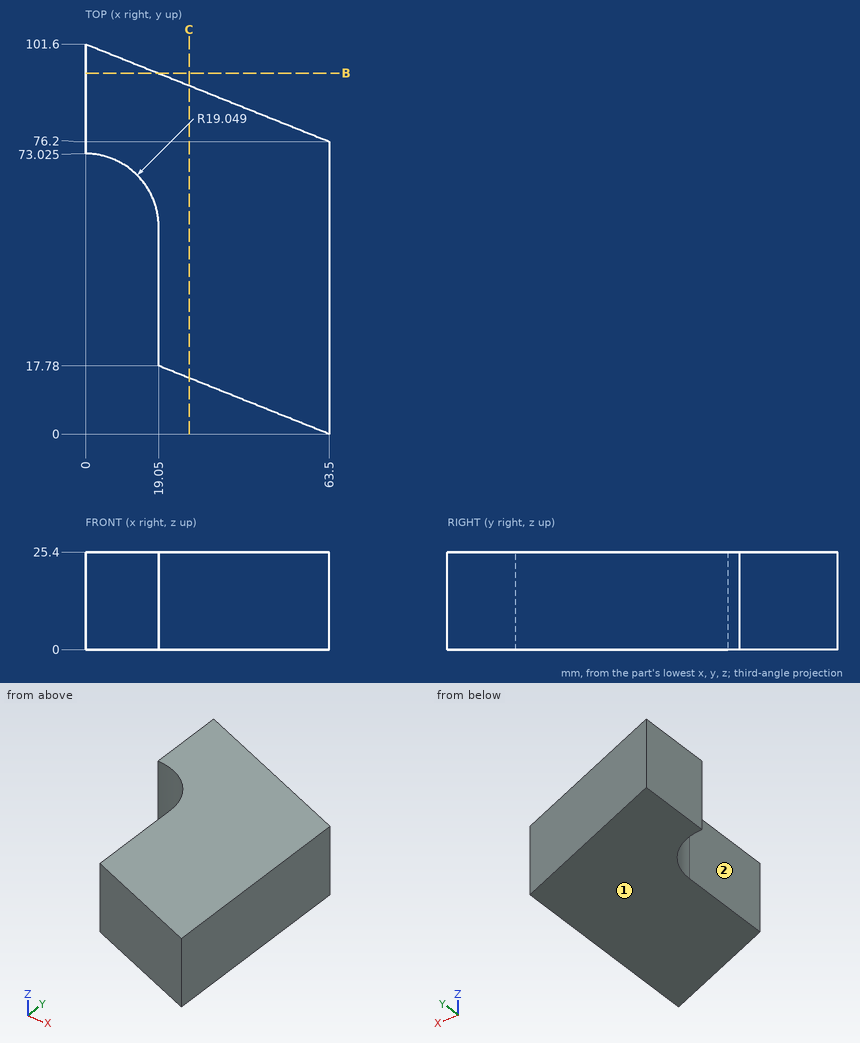
For this review, use the dimensioned drawing (mm, ordinates from the lowest corner) and the shaded views. A direction names the side the tool comes from. Coordinates: 2 decimals unless noted, no trailing zeros. Order: outer loops, then holes, each group sorted by start corner. A loop starts at its lowest first (then second) coordinate and runs counter-clockwise, first axis right, second up. Notation, with made-up numbers: M 82.5,65 L 133.5,65 A19 cw 133.5,99 Z; hole C -17.5,-27 d1. An arc over 180 degrees is marked long. Answer as a JSON object with one key per item and string values. Group by question number.
1) Add section C-C, the plane x = 27. Write out the cut boundary in (y, z).
2) Wall thickness on L1, parallel to X at y = 46, z = 2.75; L2, parallel to Y at x = 48.5, z = 2.5; L3, parallel to X at y = 61, z = 17.75: over which ranges is each line inside the solid? List them lowest first.
3) Tool access review of the marked faces 1 and 2: name each direction out of +Z, -Z, +X, -X, +Y, -Y from which nothing blocks a thin tool from reaching the whole face with its end or side.
4) Add section B-B, the plane y = 94. Write out the cut boundary in (x, z), then the cut area to 3 significant figures.
5) For pin 1 (1 mm diameter, centred on x = 8.5, z = 12.5, fed in from -Y) (1 decimal); pin 2 (12 mm diameter, centred on x = 7.5, z = 21.5, fed in from +Y); pin 3 (10 mm diameter, centred on x = 23, y = 49, fed in from -Z); pin 4 (2 mm diameter, centred on x = 30, z = 11, fed in from +Y), all flat-tipped, find the tip position at first contact; note any pin that passes through.
Computed values:
{
 "1": {"outline": "M 14.6,0 L 90.8,0 L 90.8,25.4 L 14.6,25.4 Z"},
 "2": {"L1": "x = 19.05 to 63.5", "L2": "y = 6 to 82.2", "L3": "x = 17.71 to 63.5"},
 "3": {"face 1": "-Z, +X, -X, +Y, -Y", "face 2": "+Z, -Z, -X, -Y"},
 "4": {"outline": "M 0,0 L 19,0 L 19,25.4 L 0,25.4 Z", "area": "483 mm^2"},
 "5": {"pin 1": "stops at y = 70.8", "pin 2": "stops at y = 101", "pin 3": "stops at z = 0", "pin 4": "stops at y = 90"}
}
